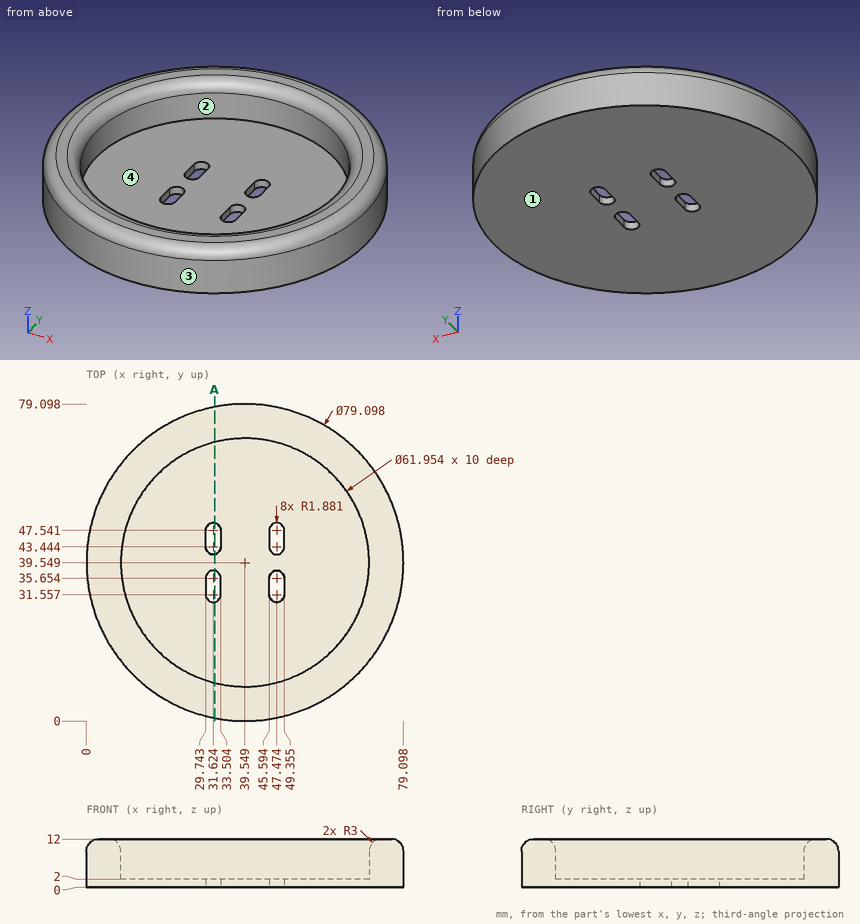
The figure shows three views and two pictorial views of one solid part (mm, origin at its lowest corner). Answer the questions. Coordinates: 2 decimals unless noted, no trailing zeros. Answer as CSV lines item,"result". Start each with the question number.
Item 1: Section A-A on x = 32 is taken. Give the number of separate pieces and of enclosed holes in the cut face, and give its area (3 significant figures).
Item 2: Determine the mould class of the marked faces 1, 2, 3 and 4 for opening direction X: released by +X, released by -X, zero draft, split by the parting line, or undercut.
Item 3: Flat-ended cylindrical pins translate along their axes: P1, Ø0.6, axis at y = 46.5, z = 0.5, coming from the +X side (1 decimal); P2, Ø6, axis at x = 46.5, z = 2, coming from the -Y side; P3, Ø1.5, axis at x = 15, z = 7.5, coming from the -Y side; P4, Ø12, axis at x = 71, y = 14.5, coming from the +Z side. Find the tip coordinate at first contact, or state that the pin passes through.
Item 4: Consider L1, parallel to X at y = 33.5, z = 1.5 (1 decimal); L2, parallel to X at y = 44, z = 1 (1 decimal); L3, parallel to Z at x = 36.5, y = 33. Determine where each line is inside the solid, lowest interval first.
Checks:
1,separate pieces,"3"
1,enclosed holes,"0"
1,area,"292 mm²"
2,face 1,"zero draft"
2,face 2,"undercut"
2,face 3,"split by the parting line"
2,face 4,"undercut"
3,P1,"stops at x = 78.5"
3,P2,"stops at y = 0.2"
3,P3,"stops at y = 7.96"
3,P4,"stops at z = 12"
4,L1,"x = 0.5 to 29.7, 33.5 to 45.6, 49.4 to 78.6"
4,L2,"x = 0.3 to 29.7, 33.5 to 45.6, 49.4 to 78.8"
4,L3,"z = 0 to 2"
